Source: CAD feature listing. Evaluate the final solid. Frame: model axes, mm. Give positions to 0.01 mm unless a question says otherwise; leave off trailing zeros. Loops run counter-clockwise (first coordinate to the right, second up) from the corner with the lowest first, then second, coordinate; pieces in that order, holes last. Notation, with made-up numbers: M 40.5,66 L 69.5,66 A17 cw 69.5,99 Z; hole C 7,-18 d4. An arc over 180 degrees is marked long. Answer in a Markdown table with one row per item.
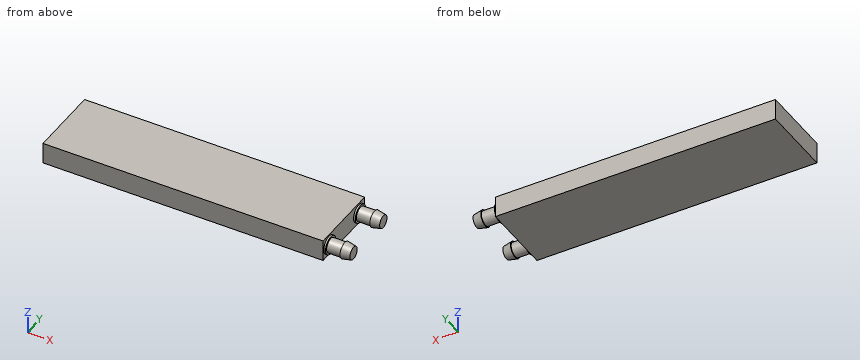
```python
from build123d import *

# Parameters (mm, degrees)
F0_W     = 161.5186
F0_H     = 41.7322
F1_DEPTH = 6.1214
F7_R     = 5.207
F7_R_2   = 4.1275
F8_DEPTH = 1.016


with BuildPart() as f1:
    # F0 (on Top) → F1 (new body, symmetric)
    with BuildSketch(Plane.XY):
        Rectangle(F0_W, F0_H)
    extrude(amount=F1_DEPTH, both=True)

    # F2 (on Top) → F3 (revolve)
    with BuildSketch(Plane.XY):
        Polygon((80.7593, -14.9479), (80.7593, -19.0754), (89.8525, -19.0754), (89.8525, -19.6723), (94.9325, -18.6309), (94.9325, -14.9479), align=None)
    revolve(axis=Axis((87.8459, -14.9479, 0), (-1, 0, 0)))

    # F4: F1 across plane


with BuildPart() as f1_1:
    add(f1.part)
    add(f1.part.mirror(Plane.XZ))

    # F7 (on face) → F8 (join)
    with BuildSketch(Plane.YZ.offset(80.7593)):
        with Locations((-14.9479, 0)):
            Circle(F7_R)
        with Locations((-14.9479, 0)):
            Circle(F7_R_2, mode=Mode.SUBTRACT)
        with Locations((14.9479, 0)):
            Circle(F7_R)
        with Locations((14.9479, 0)):
            Circle(F7_R_2, mode=Mode.SUBTRACT)
    extrude(amount=F8_DEPTH)


solid = f1_1.part
```
Q1. Section query B-B (y = 7.5). Output: boundary loops of the cut face in (x, z).
Values follow:
| item | result |
|---|---|
| outline | M -80.76,-6.12 L 80.76,-6.12 L 80.76,6.12 L -80.76,6.12 Z |
Q2. Ray query, probe 1 along X at (y, z) = (16.5, 4.5); probe 2 along X at (y, z) = (12, 4.5). Return the intervals inside material, ascending. Write a range as from..to.
Values follow:
| item | result |
|---|---|
| probe 1 | -80.76..81.78 |
| probe 2 | -80.76..80.76 |
Q3. Contact query for a flat-ended pin moving along its axis: pin 1 Ø6 at (y, z) = (0, 0.5) entering from +X. Output: stop coordinate, or through.
Values follow:
| item | result |
|---|---|
| pin 1 | x = 80.76 |
Q4. Section query A-A (z = 0). Output: boundary loops of the cut face in (x, y), plus the area to 3 significant figures.
Values follow:
| item | result |
|---|---|
| outline | M -80.76,-20.87 L 80.76,-20.87 L 80.76,-20.15 L 81.78,-20.15 L 81.78,-19.08 L 89.85,-19.08 L 89.85,-19.67 L 94.93,-18.63 L 94.93,-11.26 L 89.85,-10.22 L 89.85,-10.82 L 81.78,-10.82 L 81.78,-9.74 L 80.76,-9.74 L 80.76,9.74 L 81.78,9.74 L 81.78,10.82 L 89.85,10.82 L 89.85,10.22 L 94.93,11.26 L 94.93,18.63 L 89.85,19.67 L 89.85,19.08 L 81.78,19.08 L 81.78,20.15 L 80.76,20.15 L 80.76,20.87 L -80.76,20.87 Z |
| area | 6,980 mm^2 |
